The listing builds one solid part. Answer for the finished solid, in the listing's coordinates (mm). A direction names the side the tool comes from. Give positions to 0.01 mm unless a question says otherwise; leave off trailing zeros. Write each loop counter-clockwise with the first axis right and the second up, starting at its lowest first coordinate (ties: lowest second). Pieces come first, ordered by that corner, then holes.
```python
from build123d import *

# Parameters (mm, degrees)
SKETCH1_W                   = 38.1
SKETCH1_H                   = 12.7
SKETCH1_W_2                 = 25.4
BOSS_EXTRUDE1_DEPTH         = 6.35
F_1_4_CLEARANCE_HOLE1_D     = 6.7564
F_1_4_CLEARANCE_HOLE1_DEPTH = 12.7
BOSS_EXTRUDE2_DEPTH         = 12.7
TOP_FILLET_R                = 3.175
BOTTOM_FILLETS_R            = 1.5875
F_1_4_CLEARANCE_HOLE2_D     = 6.5278
F_1_4_CLEARANCE_HOLE2_DEPTH = 12.7
FILLET1_R                   = 6.35


with BuildPart() as part:
    # Sketch1 → Boss-Extrude1 (new body, symmetric)
    with BuildSketch(Plane(origin=(0, 0, 0), x_dir=(0, 0, -1), z_dir=(1, 0, 0))):
        Polygon((0, 139.7), (0, 0), (-215.9, 0), align=None)
        with Locations((-45.24375, -6.35)):
            Rectangle(SKETCH1_W, SKETCH1_H)
        with Locations((-177.00625, -6.35)):
            Rectangle(SKETCH1_W_2, SKETCH1_H)
    extrude(amount=BOSS_EXTRUDE1_DEPTH, both=True)

    # 1/4 Clearance Hole1
    with Locations(Plane(origin=(6.35, 0, 0), x_dir=(0, 0, -1), z_dir=(1, 0, 0))):
        with Locations((-88.9, 25.4), (-120.65, 25.4)):
            Hole(F_1_4_CLEARANCE_HOLE1_D / 2, depth=F_1_4_CLEARANCE_HOLE1_DEPTH)

    # Sketch13 → Boss-Extrude2 (add, through all)
    with BuildSketch(Plane.ZY.offset(6.35)):
        Polygon((-25.4, 156.135294118), (0, 139.7), (0, 63.5), (-25.4, 63.5), align=None)
    extrude(amount=-BOSS_EXTRUDE2_DEPTH)

    # top fillet
    top_fillet_edges = [part.edges().sort_by_distance(p)[0] for p in [
        (0, 156.135294118, -25.4),
    ]]
    fillet(top_fillet_edges, radius=TOP_FILLET_R)

    # bottom fillets
    bottom_fillets_edges = [part.edges().sort_by_distance(p)[0] for p in [
        (0, 0, 0),
        (0, 0, 26.19375),
        (0, -12.7, 26.19375),
        (0, -12.7, 64.29375),
        (0, 0, 64.29375),
        (0, 0, 164.30625),
        (0, -12.7, 164.30625),
        (0, -12.7, 189.70625),
        (0, 0, 189.70625),
        (0, 0, 215.9),
    ]]
    fillet(bottom_fillets_edges, radius=BOTTOM_FILLETS_R)

    # 1/4 Clearance Hole2
    with Locations(Plane(origin=(6.35, 0, 0), x_dir=(0, 0, -1), z_dir=(1, 0, 0))):
        with Locations((15.875, 130.175)):
            Hole(F_1_4_CLEARANCE_HOLE2_D / 2, depth=F_1_4_CLEARANCE_HOLE2_DEPTH)

    # Fillet1
    fillet1_edges = [part.edges().sort_by_distance(p)[0] for p in [
        (0, 63.5, -25.4),
        (0, 63.5, 0),
    ]]
    fillet(fillet1_edges, radius=FILLET1_R)


solid = part.part
```
Item 1: A cutting plane is placed at A-A, the plane x = 1. Count the separate pieces of the cut face and the enclosed holes in it, plus the area to 3 significant figures.
Conclusion:
separate pieces: 1
enclosed holes: 3
area: 17,900 mm2
Item 2: A cutting plane is placed at B-B, the plane z = 88.9. Give the vertices of the cut face in (x, y), plus the area to 3 significant figures.
Conclusion:
outline: (-6.35, 0) - (6.35, 0) - (6.35, 22.02) - (-6.35, 22.02) - close; (-6.35, 28.78) - (6.35, 28.78) - (6.35, 82.18) - (-6.35, 82.18) - close
area: 958 mm2
Item 3: Which of the six approach directions +Z, -Z, +X, -X, +Y, -Y give full straight-line access (tool end or side, diameter ignored) to faces 5 (the face through (-0.089, 23.344, 86.219)), 6 (the face through (0, 0, 201)), 7 (the face through (0, 30, 0)), 8 (the face through (0, -6, 164.306))?
Conclusion:
face 5: +X, -X
face 6: +Z, +X, -X, -Y
face 7: -Z, +X, -X, -Y
face 8: +X, -X, -Y
Item 4: Determine the mould class of faces 1 (the face through (-0.09, 133.41, -16.3)), 2 (the face through (0, -6, 64.294)), 3 (the face through (0, 0, 13)), 4 (the face through (0, -6, 189.706)) for opening direction Z: pulls with the +Z half, pulls with the -Z half, needs draft (parallel to the pull), parting line crosses it, or undercut.
Conclusion:
face 1: undercut
face 2: undercut
face 3: needs draft
face 4: pulls with the +Z half
Item 5: A cutting plane is placed at D-D, the plane y = 91. Give the vertices of the cut face in (x, z), plus the area to 3 significant figures.
Conclusion:
outline: (-6.35, -25.4) - (6.35, -25.4) - (6.35, 75.26) - (-6.35, 75.26) - close
area: 1,280 mm2
Item 6: Each of these flat-tipped pins is pushed along its axis until it touches: P1, Ø4, axis at x = -2, y = 26.5, coming from the -Z side; P2, Ø7.5, axis at x = 3, y = -6.5, coming from the -Z side; P3, Ø5, axis at x = 0.5, y = -6.5, coming from the +Z side. Where does it stop, or does it pass through?
Conclusion:
P1: stops at z = 0
P2: stops at z = 26.19
P3: stops at z = 189.71
Item 7: Consider probe 1 along Z at (x, y) = (-1.25, -4); probe 2 along Z at (x, y) = (3.75, 129.5); probe 3 along Y at (x, z) = (1, 88.9). Determine where each line is inside the solid, lowest interval first.
Conclusion:
probe 1: z = 26.19 to 64.29, 164.31 to 189.71
probe 2: z = -25.4 to -19.07, -12.68 to 15.76
probe 3: y = 0 to 22.02, 28.78 to 82.18
Item 8: A cutting plane is placed at C-C, the plane z = 120.65. Give the vertices of the cut face in (x, y), plus the area to 3 significant figures.
Conclusion:
outline: (-6.35, 0) - (6.35, 0) - (6.35, 22.02) - (-6.35, 22.02) - close; (-6.35, 28.78) - (6.35, 28.78) - (6.35, 61.63) - (-6.35, 61.63) - close
area: 697 mm2
